Here's the drawing with two shaded views (mm, measured from the low corner). I have some questions. Coordinates: 2 decimals unless noted, no trailing zeros. Loops run counter-clockwise (first coordinate to the right, second up) from the corner with the lowest first, then second, coordinate; pieces in that order, holes last. Notation, with made-up numbers: (34.5, 16.25) -> (68.5, 16.25) arc R37 cw to (68.5, 52.25) -> close; hole circle Ø2 at (-23.75, 3). An arc over 180 degrees is marked (long way). Answer as a JSON object with one key per item and string values. Group by question number.
1) I need wall thicknesses on probe 1 along X at (y, z) = (21.5, 8.75); probe 2 along Y at (x, z) = (13.5, 2.75) (1 decimal); probe 3 along X at (y, z) = (12.75, 1.75) (1 decimal). Which ranges of each line are inside material? Lowest first, please. Write a range as [from, to].
2) I want a section at A-A (z = 9.5). Write out the boundary of the cut face in (x, y).
3) I want a section at C-C (x = 15.5). Write out the boundary of the cut face in (y, z).
4) I'm going to push flat-ended pins straight in: pin 1 (1 mm diameter, centred on y = 20, z = 1.5, fed in from -X); pin 2 (6 mm diameter, centred on y = 9.5, z = 5.5, fed in from -X). Where does each tip first touch, or does it pass through?
5) I want a section at B-B (y = 4.5). Write out the boundary of the cut face in (x, z), then the cut area to 3 significant figures.
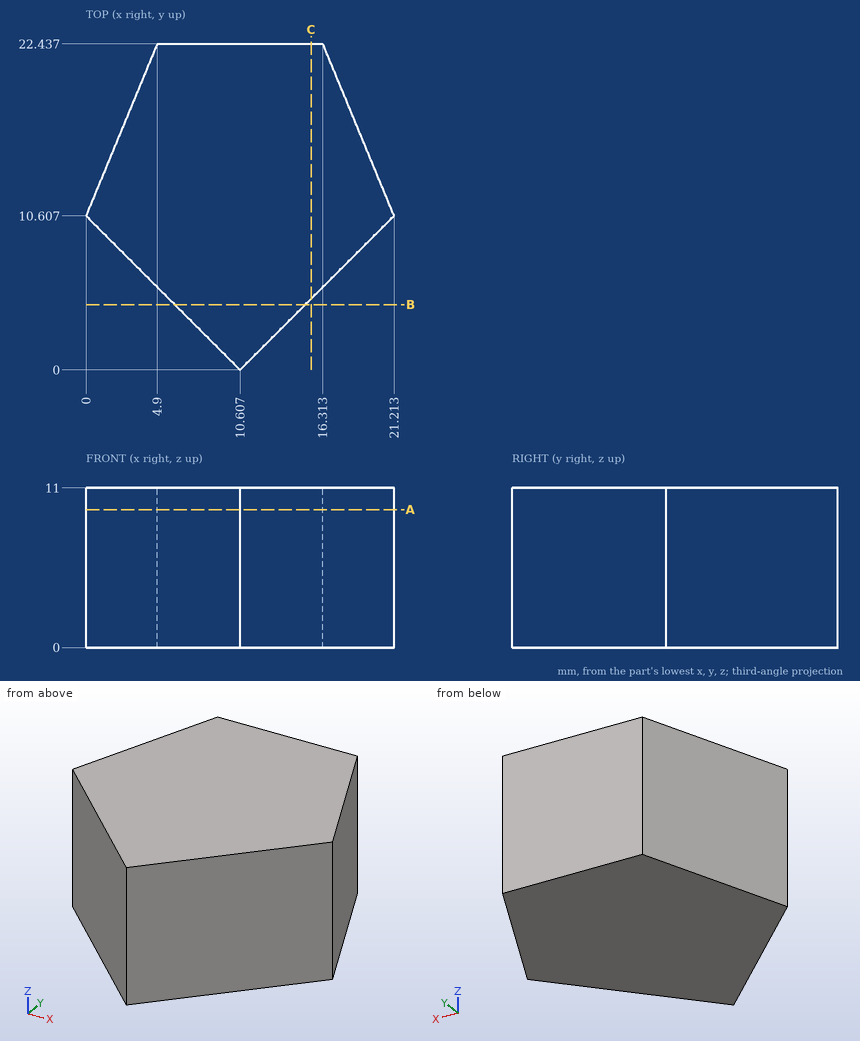
Determined:
{
 "1": {"probe 1": "[4.51, 16.7]", "probe 2": "[2.9, 22.4]", "probe 3": "[0.9, 20.3]"},
 "2": {"outline": "(0, 10.61) -> (10.61, 0) -> (21.21, 10.61) -> (16.31, 22.44) -> (4.9, 22.44) -> close"},
 "3": {"outline": "(4.89, 0) -> (22.44, 0) -> (22.44, 11) -> (4.89, 11) -> close"},
 "4": {"pin 1": "x = 3.68", "pin 2": "x = 0"},
 "5": {"outline": "(6.11, 0) -> (15.11, 0) -> (15.11, 11) -> (6.11, 11) -> close", "area": "99.0 mm^2"}
}
